Source: CAD feature listing. Evaluate the final solid. Frame: model axes, mm. A direction names the side the tool comes from. Give positions to 0.01 mm unless a question says otherwise; leave off trailing zeros. Order: outer loops, then holes, each group sorted by start corner. A loop starts at its lowest first (then second) coordinate and runs counter-clockwise, first axis right, second up. Notation, with made-up numbers: M 71.5,19 L 78.5,19 A15 ccw 78.5,32 Z; hole C 37.5,44 d5. An arc over 180 degrees is marked long. Answer as a JSON object with one key per item and string values. Group by question number.
1. Section query A-A (z = 0). Output: boundary loops of the cut face in (x, y) (3 decimals), plus the area to 3 significant figures.
2. Pin query (flat end, axial travel): P1, Ø1.5, axis at y = 2, z = 34, coming from the -X side; P2, Ø1, axis at x = 6.5, y = 1.5, coming from the +Z side; P3, Ø1.2, axis at x = 5, z = 5, coming from the +Y side; P4, Ø1, axis at y = 2.5, z = 9.5, coming from the -X side. Return the tip coordinate at first contact, or that it passes through.
3. Pull-direction query (Z, two-part tool) for faces 5 (the cylindrical face through (-9.4, 1.62, -9.43)), 6 (the cylindrical face through (-2.44, 1.58, -0.54)), 7 (the flat face through (6, 2, 10)); classes: +Z half, -Z half, draft (parallel to the pull), parting line (faces both ways), or undercut.
4. Set-up query: faces 1 (the flat face through (-6, 2, 10)), 2 (the flat face through (-5.625, 2, 0)), 3 (the flat face through (3.333, 2, 25)), 4 (the cylindrical face through (4, 2, -5)). Return all of +Z, -Z, +X, -X, +Y, -Y with unobstructed straight access to the full face (end or side cutting, diameter ignored); none if empty.
5. Section query C-C (x = 0). Output: boundary loops of the cut face in (y, z), plus the area to 3 significant figures.
6. Section query D-D (x = -7.5). Output: boundary loops of the cut face in (y, z), plus the area to 3 significant figures.
7. Material intervals for L1, parallel to X at y = 0.9, z = -5; L2, parallel to X at y = 2.45, z = -3 (3 decimals); L3, parallel to X at y = 2.05, z = 0 (3 decimals), sorted ascending. Write a range as [from, to].
from build123d import *

# Parameters (mm, degrees)
BASE_SKETCH_R       = 2.5
BOSS_EXTRUDE1_DEPTH = 3.2
FILLET1_R           = 2


with BuildPart() as part:
    # Base_Sketch → Boss-Extrude1 (new body)
    with BuildSketch(Plane(origin=(0, 0, 0), x_dir=(1, 0, 0), z_dir=(0, 1, 0))):
        with BuildLine():
            Line((-5.625, 10), (-10, 10))
            Line((-10, 10), (-10, -10))
            Line((-10, -10), (-3.333333333, -10))
            Line((-3.333333333, -10), (-3.333333333, -40))
            Line((-3.333333333, -40), (3.333333333, -40))
            Line((3.333333333, -40), (3.333333333, -10))
            Line((3.333333333, -10), (10, -10))
            Line((10, -10), (10, 10))
            Line((10, 10), (5.625, 10))
            Line((5.625, 10), (5.625, 5.78062475))
            ThreePointArc((5.625, 5.78062475), (5.901387819, 5.433012702), (6, 5))
            ThreePointArc((6, 5), (5.901387819, 4.566987298), (5.625, 4.21937525))
            Line((5.625, 4.21937525), (5.625, -4.21937525))
            ThreePointArc((5.625, -4.21937525), (5.901387819, -4.566987298), (6, -5))
            ThreePointArc((6, -5), (4.566987298, -5.901387819), (4.375, -4.21937525))
            Line((4.375, -4.21937525), (4.375, 4.21937525))
            ThreePointArc((4.375, 4.21937525), (4, 5), (4.375, 5.78062475))
            Line((4.375, 5.78062475), (4.375, 10))
            Line((4.375, 10), (-4.375, 10))
            Line((-4.375, 10), (-4.375, 5.78062475))
            ThreePointArc((-4.375, 5.78062475), (-4.098612181, 5.433012702), (-4, 5))
            ThreePointArc((-4, 5), (-4.098612181, 4.566987298), (-4.375, 4.21937525))
            Line((-4.375, 4.21937525), (-4.375, -4.21937525))
            ThreePointArc((-4.375, -4.21937525), (-4.098612181, -4.566987298), (-4, -5))
            ThreePointArc((-4, -5), (-5.433012702, -5.901387819), (-5.625, -4.21937525))
            Line((-5.625, -4.21937525), (-5.625, 4.21937525))
            ThreePointArc((-5.625, 4.21937525), (-6, 5), (-5.625, 5.78062475))
            Line((-5.625, 5.78062475), (-5.625, 10))
        make_face()
        with Locations(Location((0, 0, 0), (0, 0, 270))):
            Circle(BASE_SKETCH_R, mode=Mode.SUBTRACT)
    extrude(amount=BOSS_EXTRUDE1_DEPTH)

    # Fillet1
    fillet1_edges = [part.edges().sort_by_distance(p)[0] for p in [
        (10, 1.6, -10),
        (10, 1.6, 10),
        (-10, 1.6, 10),
        (-10, 1.6, -10),
    ]]
    fillet(fillet1_edges, radius=FILLET1_R)


solid = part.part
Answer sheet:
{
 "1": {"outline": "M -10,0 L -5.625,0 L -5.625,3.2 L -10,3.2 Z; M -4.375,0 L -2.5,0 L -2.5,3.2 L -4.375,3.2 Z; M 2.5,0 L 4.375,0 L 4.375,3.2 L 2.5,3.2 Z; M 5.625,0 L 10,0 L 10,3.2 L 5.625,3.2 Z", "area": "40.0 mm^2"},
 "2": {"P1": "x = -3.33", "P2": "z = 10", "P3": "through", "P4": "x = -9.73"},
 "3": {"face 5": "-Z half", "face 6": "undercut", "face 7": "+Z half"},
 "4": {"face 1": "+Z, -X, +Y, -Y", "face 2": "-Z, +Y, -Y", "face 3": "+Z, +X, +Y, -Y", "face 4": "+Y, -Y"},
 "5": {"outline": "M 0,-10 L 3.2,-10 L 3.2,-2.5 L 0,-2.5 Z; M 0,2.5 L 3.2,2.5 L 3.2,40 L 0,40 Z", "area": "144 mm^2"},
 "6": {"outline": "M 0,-10 L 3.2,-10 L 3.2,10 L 0,10 Z", "area": "64.0 mm^2"},
 "7": {"L1": "[-10, -6], [-4, 4], [6, 10]", "L2": "[-10, -5.625], [-4.375, 4.375], [5.625, 10]", "L3": "[-10, -5.625], [-4.375, -2.5], [2.5, 4.375], [5.625, 10]"}
}
